Autodesk Fusion 360 part; units mm, degrees
sketch "Sketch1" plane through (0, 0, 0) normal (0, 0, 1) x (1, 0, 0)
  line L0 (15, 15) -> (-15, 15)
  line L1 (-15, 15) -> (-15, -15)
  line L2 (-15, -15) -> (15, -15)
  line L3 (15, -15) -> (15, 15)
  line L4 (15, 15) -> (-15, -15) construction
  line L5 (-15, 15) -> (15, -15) construction
  dimension "d1" = 30
  dimension "d2" = 30
extrude "Extrude1" add sketch "Sketch1" along normal blind 3
sketch "Sketch2" plane through (0, 0, 3) normal (0, 0, 1) x (-1, 0, 0)
  line L0 (-15, 15) -> (-15, -15)
  line L1 (-15, -15) -> (15, -15)
  line L2 (15, -15) -> (15, 15)
  line L3 (15, 15) -> (-15, 15)
  circle A0 centre (0, 0) radius 2
  dimension "d5" = 4
extrude "Extrude2" add sketch "Sketch2" along normal blind 8.5 contours A0
sketch "Sketch3" plane through (0, 0, 11.5) normal (0, 0, 1) x (-1, 0, 0)
  circle A0 centre (0, 0) radius 2
  circle A1 centre (0, 0) radius 1.35
  dimension "d8" = 2.7
extrude "Extrude3" cut sketch "Sketch3" against normal blind 1 contours A1
sketch "Sketch4" plane through (0, 0, 3) normal (0, 0, 1) x (-1, 0, 0)
  circle A0 centre (0, 0) radius 2
  line L0 (-15, 15) -> (-15, -15)
  line L1 (-15, -15) -> (15, -15)
  line L2 (15, -15) -> (15, 15)
  line L3 (15, 15) -> (-15, 15)
  line L4 (3.06, -5.3) -> (6.1199, 0)
  line L5 (6.1199, 0) -> (3.06, 5.3)
  line L6 (3.06, 5.3) -> (-3.06, 5.3)
  line L7 (-3.06, 5.3) -> (-6.1199, 0)
  line L8 (-6.1199, 0) -> (-3.06, -5.3)
  line L9 (-3.06, -5.3) -> (3.06, -5.3)
  line L10 (9.2953, 0) -> (4.6477, 8.05)
  line L11 (4.6477, 8.05) -> (-4.6477, 8.05)
  line L12 (-4.6477, 8.05) -> (-9.2953, 0)
  line L13 (-9.2953, 0) -> (-4.6477, -8.05)
  line L14 (-4.6477, -8.05) -> (4.6477, -8.05)
  line L15 (4.6477, -8.05) -> (9.2953, 0)
  line L16 (15, 3.5) -> (-15, 3.5)
  dimension "d11" = 10.5
  dimension "d12" = 2.75
  dimension "d13" = 3.5
extrude "Extrude4" add sketch "Sketch4" along normal blind 20 contours L4 L5 L7 L8 L9 L10 L12 L13 L14 L15 L16
chamfer "Chamfer1" distance 1 angle 45 2 edges at (4.0992, -3.5, 13) (-4.0992, -3.5, 13)
chamfer "Chamfer2" distance 2 angle 45 3 edges at (6.9715, 4.025, 3) (0, 8.05, 3) (-6.9715, 4.025, 3)
chamfer "Chamfer2" distance 2 angle 45 2 edges at (8.285, -1.75, 3) (-8.285, -1.75, 3)
chamfer "Chamfer2" distance 0.5 angle 45 1 edges at (1.8647, -0.7232, 3)
Model file for the job. Use its own axes, mm. A direction names the side the tool comes from. Coordinates: 2 decimals unless noted, no trailing zeros. Loops run counter-clockwise (first coordinate to the right, second up) from the corner with the lowest first, then second, coordinate; pieces in that order, holes last. Notation, with made-up numbers: M -6,73 L 33,73 A29 ccw 33,105 Z; hole C -29.5,-4 d9. An arc over 180 degrees is marked long. Use CSV: the item, a comma, the result in double quotes. Start each with the question number.
1. Tool access for faces 5 (the flat face through (4.846, -3.061, 13.14)), 6 (the flat face through (6, -3.5, 13)), 7 (the flat face through (7.004, 3.969, 13.874)), 8 (the flat face through (0, 0, 0)), 9 (the flat face through (0, -3, 3)): list every direction of +Z, -Z, +X, -X, +Y, -Y with a clear straight run to the whole face (end or side of a thin tool).
2. Band-saw the part on C-C, the plane y = -4.75. List the corners of the cut face in (x, z), then the cut area to 3 significant figures.
3. Band-saw the part on B-B, the plane z = 13.25. List the corners of the cut face in (x, y), then the cut area to 3 significant figures.
4. Band-saw the part on D-D, the plane x = -3.5. List the corners of the cut face in (y, z), then the cut area to 3 significant figures.
5. Band-saw the part on A-A, the plane x = 0. List the corners of the cut face in (y, z).
6. Two-plate mould, pull along Y, no slides. Class faces 1 (the flat face through (0, 8.05, 14)), 2 (the flat face through (0, 5.3, 13)), 3 (the flat face through (0, 6, 23)), 4 (the flat face through (8.271, -1.774, 13.874)): pulls with the +Y half, pulls with the -Y half, needs draft (parallel to the pull), parting line crosses it, or undercut.
7. Probe probe 1 along X at (y, z) = (0, 11); probe 2 along Y at (x, z) = (0, 11.2); probe 3 along Z at (x, y) = (2.5, 11.25). List the from-to ranges inside material, lowest first. Write a range as [from, to].
8. Flat gauge pins, fed straight in: pin 1 (7.5 mm diameter, centred on x = -2, z = 16, fed in from +Y); pin 2 (3 mm diameter, centred on x = 0, z = 15, fed in from -Y); pin 3 (3 mm diameter, centred on y = 9, z = 12, fed in from -X). Where does each tip first touch, or does it go through?
Entries:
1,face 5,"+Z, -Y"
1,face 6,"+Z, +X, -X, -Y"
1,face 7,"+Z, +X, +Y"
1,face 8,"-Z, +X, -X, +Y, -Y"
1,face 9,"+Z"
2,outline,"M -15,0 L 15,0 L 15,3 L -15,3 Z"
2,area,"90.0 mm2"
3,outline,"M -9.3,0 L -7.27,-3.5 L -5.1,-3.5 L -4.6,-2.63 L -6.12,0 L -3.06,5.3 L 3.06,5.3 L 6.12,0 L 4.6,-2.63 L 5.1,-3.5 L 7.27,-3.5 L 9.3,0 L 4.65,8.05 L -4.65,8.05 Z"
3,area,"84.9 mm2"
4,outline,"M -15,0 L 15,0 L 15,3 L 10.05,3 L 8.05,5 L 8.05,23 L 4.54,23 L 4.54,3 L -15,3 Z"
4,area,"162 mm2"
5,outline,"M -15,0 L 15,0 L 15,3 L 10.05,3 L 8.05,5 L 8.05,23 L 5.3,23 L 5.3,3 L 2.5,3 L 2,3.5 L 2,11.5 L 1.35,11.5 L 1.35,10.5 L -1.35,10.5 L -1.35,11.5 L -2,11.5 L -2,3.5 L -2.5,3 L -15,3 Z"
6,face 1,"pulls with the +Y half"
6,face 2,"undercut"
6,face 3,"needs draft"
6,face 4,"pulls with the -Y half"
7,probe 1,"x = [-9.3, -6.12], [-2, -1.35], [1.35, 2], [6.12, 9.3]"
7,probe 2,"y = [-2, -1.35], [1.35, 2], [5.3, 8.05]"
7,probe 3,"z = [0, 3]"
8,pin 1,"stops at y = 8.05"
8,pin 2,"stops at y = 5.3"
8,pin 3,"stops at x = -4.97"
